Read the model definition and answer for the solid it produces. Units are mm, in the model's axes. Give positions to 0.01 mm unless a question says otherwise; leave off trailing zeros. Write each loop counter-clockwise with the first axis right and the second up, starting at its lowest first coordinate (ties: lowest second). Pieces come first, ordered by that corner, then holes. Notation, with made-up numbers: M 63,4.5 L 82,4.5 A30 cw 82,42.5 Z; hole C 19,-23.5 d11. An arc over 180 degrees is marked long. Write each question's results on one line, items separated by ' | '. Start each with the question number.
Autodesk Inventor part; units mm, degrees
ref_plane "YZ Plane" through (0, 0, 0) normal (1, 0, 0) x (0, 1, 0)
ref_plane "XZ Plane" through (0, 0, 0) normal (0, 1, 0) x (-1, 0, 0)
ref_plane "XY Plane" through (0, 0, 0) normal (0, 0, 1) x (1, 0, 0)
sketch "Sketch1" plane through (0, 0, 0) normal (0, 0, 1) x (1, 0, 0)
  line L0 (-27.25, 33) -> (27.25, 33)
  line L1 (27.25, 33) -> (27.25, -33)
  line L2 (27.25, -33) -> (-27.25, -33)
  line L3 (-27.25, -33) -> (-27.25, 33)
  point P0 (0, 0)
  point P1 (0, 33)
  point P2 (-27.25, 0)
  dimension "d0" = 54.5
  dimension "d1" = 66
extrude "Extrusion1" add sketch "Sketch1" along normal blind 8
sketch "Sketch2" plane through (0, 0, 8) normal (0, 0, 1) x (1, 0, 0)
  circle A0 centre (6.25, 10) radius 7.5
  line L0 (27.25, 33) -> (-27.25, 33)
  line L1 (-27.25, 33) -> (-27.25, -33)
  line L2 (27.25, -33) -> (27.25, 33)
  line L3 (21.75, -5.5) -> (-9.25, -5.5) construction
  line L4 (-9.25, -5.5) -> (-9.25, 25.5) construction
  line L5 (-9.25, 25.5) -> (21.75, 25.5) construction
  line L6 (21.75, 25.5) -> (21.75, -5.5) construction
  line L7 (21.75, -5.5) -> (-9.25, 25.5) construction
  line L8 (-9.25, -5.5) -> (21.75, 25.5) construction
  circle A1 centre (-9.25, -5.5) radius 1.75
  circle A2 centre (-9.25, 25.5) radius 1.75
  circle A3 centre (21.75, 25.5) radius 1.75
  circle A4 centre (21.75, -5.5) radius 1.75
  point P0 (0, 33)
  point P1 (-27.25, 0)
  dimension "d17" = 15
  dimension "d19" = 21
  dimension "d20" = 23
  dimension "d22" = 31
  dimension "d23" = 3.5
extrude "Extrusion2" cut sketch "Sketch2" against normal through all
sketch "Sketch4" plane through (0, 0, 8) normal (0, 0, 1) x (1, 0, 0)
  circle A0 centre (8.2191, -13) radius 4
  line L0 (-27.25, -33) -> (27.25, -33)
  line L1 (27.25, -33) -> (27.25, 33)
  point P0 (0, 0)
  dimension "d24" = 8
  dimension "d25" = 20
  dimension "d26" = 19.0309
extrude "Extrusion4" cut sketch "Sketch4" against normal through all
sketch "Sketch5" plane through (0, 0, 8) normal (0, 0, 1) x (1, 0, 0)
  line L0 (-27.25, 33) -> (-27.25, -33)
  point P0 (0, 0)
  point P1 (-23.25, 0)
  point P2 (-23.25, -23)
  point P3 (-23.25, 23)
  dimension "d29" = 4
  dimension "d30" = 23
  dimension "d31" = 23
hole "Hole1" at (-23.25, 0, 8) at (-23.25, -23, 8) at (-23.25, 23, 8) direction (0, 0, -1) diameter 4.5 end through all
properties part number "0005-10-007Suport nema"
Item 1: Section A-A, the plane y = -13 is taken. Determine the outline of the cut face in (x, z), then the cut area to 3 significant figures.
Item 2: Determine the mould class of faces 1 (the flat face through (-27.25, 0, 4)), 2 (the flat face through (27.25, 0, 4)), 3 (the flat face through (0, -33, 4)), 4 (the cylindrical face through (4.62, 2.68, 4.06)) for opening direction X: +X half, -X half, draft (parallel to the pull), parting line (faces both ways), or undercut.
Item 3: Section B-B, the plane x = -9.25 is taken. Determine the outline of the cut face in (y, z).
Item 4: Section D-D, the plane x = 0.5 is taken. Determine the outline of the cut face in (y, z).
Item 5: Given P1, Ø4.5, axis at x = 21.75, y = -5.5, coming from the -Z side, flat-ended and moving along its own axis, determine where the tip first touches the part or whether it passes through.
Item 6: Section C-C, the plane z = 1.25 is taken. Give the number of separate pieces and of enclosed holes in the cut face, then the cut area to 3 significant figures.
Item 7: Straight lines are drawn through the part: line 1 (Y direction, x = -23.25, z = 5.5); line 2 (Y direction, x = 21.75, z = 3.5); line 3 (Y direction, x = -8, z = 6.25). For each, find the intervals that lie inside material, in ascending order.
Worked out:
1) outline: M -27.25,0 L 4.22,0 L 4.22,8 L -27.25,8 Z; M 12.22,0 L 27.25,0 L 27.25,8 L 12.22,8 Z | area: 372 mm²
2) face 1: -X half | face 2: +X half | face 3: draft | face 4: undercut
3) outline: M -33,0 L -7.25,0 L -7.25,8 L -33,8 Z; M -3.75,0 L 23.75,0 L 23.75,8 L -3.75,8 Z; M 27.25,0 L 33,0 L 33,8 L 27.25,8 Z
4) outline: M -33,0 L 5.18,0 L 5.18,8 L -33,8 Z; M 14.82,0 L 33,0 L 33,8 L 14.82,8 Z
5) P1: stops at z = 0
6) separate pieces: 1 | enclosed holes: 9 | area: 3,280 mm²
7) line 1: y = -33 to -25.25, -20.75 to -2.25, 2.25 to 20.75, 25.25 to 33 | line 2: y = -33 to -7.25, -3.75 to 23.75, 27.25 to 33 | line 3: y = -33 to -6.72, -4.28 to 24.28, 26.72 to 33
